For this review, take the finished solid that the model builds, in its own axes (mm). A direction names the side the tool comes from. Give positions to 0.01 mm unless a question says otherwise; leave off trailing zeros. Write each loop counter-clockwise with the first axis right and the second up, starting at its lowest first coordinate (ties: lowest second). Pieces come first, ordered by that corner, then holes. Notation, with made-up numbers: M 0.25,2 L 33.25,2 A25 cw 33.25,19 Z; hole C 21.25,-4.5 d5. An arc over 180 degrees is marked long. Write item = value, one per line.
```python
from build123d import *

# Parameters (mm, degrees)
F1_DEPTH = 25.4
F3_D     = 6.35
F5_D     = 6.35


# Not quite as in the source:
# - a feature names something its author has since deleted; it is built from what else it names


with BuildPart() as f1:
    # F0 (on Right) → F1 (new body)
    with BuildSketch(Plane.YZ):
        Polygon((14.3006006256, -31.3609689474), (-48.9231087267, -31.3609689474), (-48.9231087267, -57.2024062276), (41.6473634541, -57.2024062276), (41.6473634541, 39.3893681467), (14.3006006256, 39.3893681467), align=None)
    extrude(amount=F1_DEPTH)

    # F3 (through all)
    with Locations(Plane.XY.offset(-31.3609689474)):
        with Locations((14.0417637303, -30.5415708572)):
            Hole(F3_D / 2)

    # F5 (through all)
    with Locations(Plane.XY.offset(-31.3609689474)):
        with Locations((12.3347630724, 0)):
            Hole(F5_D / 2)


solid = f1.part
```
1. For line 1 along Z through (x, y) = (2.25, -9); line 2 along Y through (x, z) = (11, 1), list the stretches that pass through material, from the lowest coordinate up. Write a range as from..to.
Responses:
line_1 = -57.2..-31.36
line_2 = 14.3..41.65
2. The part is to be moulded in two halves that separate along Y. For faces 3 (the face through (25.4, 16, -19)), 4 (the face through (14.854, -1.932, -44.463)), 5 (the face through (13, 14.301, 5)), say which applies: +Y half, -Y half, draft (parallel to the pull), parting line (faces both ways), or undercut.
Responses:
face_3 = draft
face_4 = undercut
face_5 = -Y half
3. We need section A-A, the plane y = 0. Write out the cut boundary in (x, z).
Responses:
outline = M 0,-57.2 L 9.16,-57.2 L 9.16,-31.36 L 0,-31.36 Z; M 15.51,-57.2 L 25.4,-57.2 L 25.4,-31.36 L 15.51,-31.36 Z
4. Machinability: for faces 1 (the face through (16.561, -32.474, -44.463)), 2 (the face through (13, -17, -31.361)), which of the approach directions +Z, -Z, +X, -X, +Y, -Y give a long, thin tool a straight path to every point of the face, cutting with its end or side? Answer none if there is none.
Responses:
face_1 = +Z, -Z
face_2 = +Z, +X, -X, -Y
5. Insertion check: P1, Ø7.5, axis at x = 12.33, y = 0, coming from the +Z side; P2, Ø7.5, axis at x = 18.5, z = -7.5, coming from the -Y side. Each pin has a flat end and moves straight along its axis. Give the tip position at first contact, or say it passes through.
Responses:
P1 = -31.36
P2 = 14.3
6. We need section B-B, the plane x = 7.75. Write out the cut boundary in (y, z).
Responses:
outline = M -48.92,-57.2 L 41.65,-57.2 L 41.65,39.39 L 14.3,39.39 L 14.3,-31.36 L -48.92,-31.36 Z
7. We need section C-C, the plane z = -11. Write out the cut boundary in (x, y).
Responses:
outline = M 0,14.3 L 25.4,14.3 L 25.4,41.65 L 0,41.65 Z
